from build123d import *

# Parameters (mm, degrees)
BOSS_EXTRUDE1_DEPTH                                 = 5
CUT_EXTRUDE1_REACH                                  = 7
SKETCH2_R                                           = 6.4897
SKETCH3_W                                           = 3
SKETCH3_H                                           = 3
BOSS_EXTRUDE2_DEPTH                                 = 6
CSK_FOR_M2_COUNTERSUNK_FLAT_HEAD_SCREW1_D           = 2.4
CSK_FOR_M2_COUNTERSUNK_FLAT_HEAD_SCREW1_DEPTH       = 5.2
CSK_FOR_M2_COUNTERSUNK_FLAT_HEAD_SCREW1_CSINK_D     = 5.4
CSK_FOR_M2_COUNTERSUNK_FLAT_HEAD_SCREW1_CSINK_ANGLE = 90
CSK_FOR_M2_COUNTERSUNK_FLAT_HEAD_SCREW1_TIP         = 0.721032743
CUT_EXTRUDE2_DEPTH                                  = 2.5
FILLET1_R                                           = 3
M2_TAPPED_HOLE1_D                                   = 1.6
M2_TAPPED_HOLE1_DEPTH                               = 2.5


with BuildPart() as part:
    # Sketch1 → Boss-Extrude1 (new body)
    with BuildSketch(Plane(origin=(0, 0, 0), x_dir=(1, 0, 0), z_dir=(0, 1, 0))):
        Polygon((-15, 0), (15, 0), (15, 35), (13.807692308, 50.5), (-13.807692308, 50.5), (-15, 35), align=None)
    extrude(amount=BOSS_EXTRUDE1_DEPTH)

    # Sketch2 → Cut-Extrude1 (cut, up to next)
    with BuildSketch(Plane(origin=(0, 5, 0), x_dir=(1, 0, 0), z_dir=(0, 1, 0)), mode=Mode.PRIVATE) as cut_extrude1_sk1:
        with Locations((0, 35)):
            Circle(SKETCH2_R)
    cut_extrude1_tool1 = extrude(cut_extrude1_sk1.sketch, amount=-CUT_EXTRUDE1_REACH, mode=Mode.PRIVATE) & part.part
    add(cut_extrude1_tool1.solids().sort_by_distance((0, 5, -35))[0], mode=Mode.SUBTRACT)

    # Sketch3 → Boss-Extrude2 (add)
    with BuildSketch(Plane(origin=(0, 5, 0), x_dir=(1, 0, 0), z_dir=(0, 1, 0))):
        with Locations((0, 4)):
            Rectangle(SKETCH3_W, SKETCH3_H)
    extrude(amount=BOSS_EXTRUDE2_DEPTH)

    # CSK for M2 Countersunk Flat Head Screw1
    with Locations(Plane(origin=(0, 0, 0), x_dir=(-1, 0, 0), z_dir=(0, -1, 0))):
        with Locations((-10, 4), (10, 4), (0, 11)):
            CounterSinkHole(CSK_FOR_M2_COUNTERSUNK_FLAT_HEAD_SCREW1_D / 2, CSK_FOR_M2_COUNTERSUNK_FLAT_HEAD_SCREW1_CSINK_D / 2, depth=CSK_FOR_M2_COUNTERSUNK_FLAT_HEAD_SCREW1_DEPTH, counter_sink_angle=CSK_FOR_M2_COUNTERSUNK_FLAT_HEAD_SCREW1_CSINK_ANGLE)
            with Locations((0, 0, -(CSK_FOR_M2_COUNTERSUNK_FLAT_HEAD_SCREW1_DEPTH + CSK_FOR_M2_COUNTERSUNK_FLAT_HEAD_SCREW1_TIP / 2))):  # 118° drill point
                Cone(0, CSK_FOR_M2_COUNTERSUNK_FLAT_HEAD_SCREW1_D / 2, CSK_FOR_M2_COUNTERSUNK_FLAT_HEAD_SCREW1_TIP, mode=Mode.SUBTRACT)

    # Sketch6 → Cut-Extrude2 (cut)
    with BuildSketch(Plane.XZ):
        with BuildLine():
            Line((-10.5, -48), (10.5, -48))
            ThreePointArc((10.5, -48), (12.267766953, -47.267766953), (13, -45.5))
            Line((13, -45.5), (13, -24.5))
            ThreePointArc((13, -24.5), (12.267766953, -22.732233047), (10.5, -22))
            Line((10.5, -22), (-10.5, -22))
            ThreePointArc((-10.5, -22), (-12.267766953, -22.732233047), (-13, -24.5))
            Line((-13, -24.5), (-13, -45.5))
            ThreePointArc((-13, -45.5), (-12.267766953, -47.267766953), (-10.5, -48))
        make_face()
    extrude(amount=-CUT_EXTRUDE2_DEPTH, mode=Mode.SUBTRACT)

    # Fillet1
    fillet1_edges = [part.edges().sort_by_distance(p)[0] for p in [
        (-13.807692308, 2.5, -50.5),
        (13.807692308, 2.5, -50.5),
    ]]
    fillet(fillet1_edges, radius=FILLET1_R)

    # M2 Tapped Hole1
    with Locations(Plane(origin=(0, 2.5, 0), x_dir=(-1, 0, 0), z_dir=(0, -1, 0))):
        with Locations((9.5, 25.5), (9.5, 44.5), (-9.5, 44.5), (-9.5, 25.5)):
            Hole(M2_TAPPED_HOLE1_D / 2, depth=M2_TAPPED_HOLE1_DEPTH)


solid = part.part
For this review, take the finished solid that the model builds, in its own axes (mm). A direction names the side the tool comes from. Round coordinates to 2 decimals unless told otherwise and drop trailing zeros. Write each loop counter-clockwise with the first axis right and the second up, starting at its lowest first coordinate (ties: lowest second). Pieces come first, ordered by that corner, then holes. Notation, with made-up numbers: (19, 69.25) - (62, 69.25) arc R19 ccw to (62, 77.25) - close; hole circle Ø3 at (-28, 22.25). An arc over 180 degrees is marked (long way). Use a Markdown table: item, result.
Q1. Clearance check with flat-ended pins moving along their axes: pin 1 (2 mm diameter, centred on x = 11.5, z = -36, fed in from -Y); pin 2 (1.5 mm diameter, centred on x = 0, y = 7, fed in from -Z); pin 3 (0.8 mm diameter, centred on y = 0.5, z = -38, fed in from +X). State where each tip first meets the part, or that it passes through.
Derived:
| item | result |
|---|---|
| pin 1 | stops at y = 2.5 |
| pin 2 | stops at z = -5.5 |
| pin 3 | stops at x = 14.8 |
Q2. We need section C-C (y = 0.75). Give the boundary of the cut face in (x, z).
Derived:
| item | result |
|---|---|
| outline | (-15, -35) - (-14.02, -47.73) arc R3 ccw to (-11.03, -50.5) - (11.03, -50.5) arc R3 ccw to (14.02, -47.73) - (15, -35) - (15, 0) - (-15, 0) - close; hole (-13, -45.5) arc R2.5 ccw to (-10.5, -48) - (10.5, -48) arc R2.5 ccw to (13, -45.5) - (13, -24.5) arc R2.5 ccw to (10.5, -22) - (-10.5, -22) arc R2.5 ccw to (-13, -24.5) - close; hole circle Ø3.9 at (-10, -4); hole circle Ø3.9 at (0, -11); hole circle Ø3.9 at (10, -4) |
Q3. Wall thickness on line 1 along Z through (x, y) = (0, 3.15); line 2 along Z through (x, y) = (10, 2.95); line 3 along X through (y, z) = (3.65, -35): over which ranges is each line inside the solid? List them lowest first.
Derived:
| item | result |
|---|---|
| line 1 | z = -50.5 to -41.49, -28.51 to -12.2, -9.8 to 0 |
| line 2 | z = -50.5 to -45.12, -43.88 to -26.12, -24.88 to -5.2, -2.8 to 0 |
| line 3 | x = -15 to -6.49, 6.49 to 15 |
Q4. We need section B-B (x = 0). Give the boundary of the cut face in (y, z), plus the area to 3 significant figures.
Derived:
| item | result |
|---|---|
| outline | (0, -50.5) - (5, -50.5) - (5, -41.49) - (2.5, -41.49) - (2.5, -48) - (0, -48) - close; (0, -22) - (2.5, -22) - (2.5, -28.51) - (5, -28.51) - (5, -12.2) - (1.5, -12.2) - (0, -13.7) - close; (0, -8.3) - (1.5, -9.8) - (5, -9.8) - (5, -5.5) - (11, -5.5) - (11, -2.5) - (5, -2.5) - (5, 0) - (0, 0) - close |
| area | 159 mm2 |
Q5. We need section D-D (z = -36). Give the boundary of the cut face in (x, y), plus the area to 3 significant figures.
Derived:
| item | result |
|---|---|
| outline | (-14.92, 0) - (-13, 0) - (-13, 2.5) - (-6.41, 2.5) - (-6.41, 5) - (-14.92, 5) - close; (6.41, 2.5) - (13, 2.5) - (13, 0) - (14.92, 0) - (14.92, 5) - (6.41, 5) - close |
| area | 52.2 mm2 |
Q6. We need section A-A (z = -4). Give the boundary of the cut face in (x, y), plus the area to 4 significant figures.
Derived:
| item | result |
|---|---|
| outline | (-15, 0) - (-12.7, 0) - (-11.2, 1.5) - (-11.2, 5) - (-15, 5) - close; (-8.8, 1.5) - (-7.3, 0) - (7.3, 0) - (8.8, 1.5) - (8.8, 5) - (1.5, 5) - (1.5, 11) - (-1.5, 11) - (-1.5, 5) - (-8.8, 5) - close; (11.2, 1.5) - (12.7, 0) - (15, 0) - (15, 5) - (11.2, 5) - close |
| area | 139.5 mm2 |
Q7. Machinability: for faces 1 (the flat face through (0, 8, -5.5)), 2 (the flat face through (0, 8, -2.5)), 3 (the cylindrical face through (12.287, 1.232, -22.752)), which of the approach directions +Z, -Z, +X, -X, +Y, -Y give a long, thin tool a straight path to every point of the face, cutting with its end or side? Answer none if there is none.
Derived:
| item | result |
|---|---|
| face 1 | -Z, +X, -X, +Y |
| face 2 | +Z, +X, -X, +Y |
| face 3 | -Y |
